For this review, take the finished solid that the model builds, in its own axes (mm). A direction names the side the tool comes from. Coordinates: 2 decimals unless noted, no trailing zeros. Loops run counter-clockwise (first coordinate to the right, second up) from the corner with the lowest first, then second, coordinate; pieces in that order, holes last. Notation, with made-up numbers: (-5, 22.25) - (12, 22.25) arc R11 cw to (12, 43.25) - close; hole circle Ø2 at (-16.75, 75). An arc over 180 degrees is marked (long way). Answer as a JSON object with one key per item and string values. Group by question number.
Item 1: Clearance check with flat-ended pins moving along their axes: pin 1 (1.8 mm diameter, centred on y = -4.5, z = -6, fed in from -X); pin 2 (3 mm diameter, centred on y = -2.5, z = -2.5, fed in from +X); pin 3 (1.5 mm diameter, centred on y = -2.5, z = -10.5, fed in from -X). State where each tip first meets the part, or that it passes through.
Item 2: Tool access review of faces 5 (the cylindrical face through (6.47, -3.46, 11.38)), 6 (the flat face through (2.5, -3, -2)): name each direction out of +Z, -Z, +X, -X, +Y, -Y from which nothing blocks a thin tool from reaching the whole face with its end or side.
Item 3: We need section B-B (x = 1.5). State how many separate pieces and enclosed holes the cut face has, then the cut area to 3 significant figures.
Item 4: We need section A-A (z = 1). Give the boundary of the cut face in (x, y), then the cut area to 3 significant figures.
Item 5: To check wall thickness, follow line 1 (X direction, y = -2, z = 10.75); line 2 (Z direction, x = -1.5, y = -1.5); line 3 (X direction, y = -2.75, z = 8). State the ranges of each line that lie inside material, in increasing order.
Item 6: Mouldability with a two-part tool opening along Z and no side actions: class faces 1 (the cylindrical face through (0.03, -1, -11.45)), 2 (the cylindrical face through (-6.47, -3.46, 11.38)), 3 (the cylindrical face through (-0.03, -2.96, -11.44)), 4 (the flat face through (-2.5, -3, -2)) as released by +Z, released by -Z, zero draft, split by the parting line, or undercut.
from build123d import *

# Parameters (mm, degrees)
F0_W         = 5
F0_H         = 17
F1_DEPTH     = 7
F3_D         = 5
F4_T1_DEPTH  = 29.5
F5_R         = 3.49999
F6_R         = 3
F7_T1_DEPTH  = 10.7715938526
F7_T3_DEPTH  = 7
F7_T5_DEPTH  = 2e-05
F7_T16_ANGLE = 74.5339900582
F7_T18_ANGLE = 117.281460121
F7_T20_ANGLE = 132.7531885059
F7_T22_ANGLE = 74.5339900582
F7_T24_ANGLE = 117.281460121
F7_T26_ANGLE = 132.7531885059
F7_T28_ANGLE = 90
F7_T30_ANGLE = 90
F7_T34_ANGLE = 74.5339900582
F7_T36_ANGLE = 90
F7_T38_ANGLE = 117.281460121
F7_T40_ANGLE = 90
F7_T44_ANGLE = 132.7531885059
F7_T46_ANGLE = 74.5339900582
F7_T48_ANGLE = 117.281460121
F7_T50_ANGLE = 132.7531885059


# Not quite as in the source:
# - a fillet or chamfer that OpenCascade refuses, or shapes differently, is made with other operations: its cross-section is extruded or revolved along the edge and cut away or added
# - two fillets or chamfers of one size are made in one step
# - a fillet or chamfer is up to 0.001 mm smaller than in the source, because OpenCascade refuses the exact size


with BuildPart() as f1:
    # F0 (on Front) → F1 (new body)
    with BuildSketch(Plane.XZ):
        with BuildLine():
            Line((8, 12.5), (2.5, 12.5))
            Line((2.5, 12.5), (2.5, 11.0980762114))
            ThreePointArc((2.5, 11.0980762114), (5.5, 11.0980762114), (7, 8.5))
            ThreePointArc((7, 8.5), (5.5, 5.9019237886), (2.5, 5.9019237886))
            Line((2.5, 5.9019237886), (2.5, 4.5))
            Line((2.5, 4.5), (8, 4.5))
            Line((8, 4.5), (8, 12.5))
        make_face()
        with BuildLine():
            Line((-2.5, 11.0980762114), (-2.5, 12.5))
            Line((-2.5, 12.5), (-8, 12.5))
            Line((-8, 12.5), (-8, 4.5))
            Line((-8, 4.5), (-2.5, 4.5))
            Line((-2.5, 4.5), (-2.5, 5.9019237886))
            ThreePointArc((-2.5, 5.9019237886), (-7, 8.5), (-2.5, 11.0980762114))
        make_face()
        with BuildLine():
            Line((2.5, 11.0980762114), (2.5, 12.5))
            Line((2.5, 12.5), (-2.5, 12.5))
            Line((-2.5, 12.5), (-2.5, 11.0980762114))
            ThreePointArc((-2.5, 11.0980762114), (-1.4019237886, 10), (-1, 8.5))
            ThreePointArc((-1, 8.5), (-1.4019237886, 7), (-2.5, 5.9019237886))
            Line((-2.5, 5.9019237886), (-2.5, 4.5))
            Line((-2.5, 4.5), (2.5, 4.5))
            Line((2.5, 4.5), (2.5, 5.9019237886))
            ThreePointArc((2.5, 5.9019237886), (1, 8.5), (2.5, 11.0980762114))
        make_face()
        with Locations((0, -4)):
            Rectangle(F0_W, F0_H)
    extrude(amount=F1_DEPTH)

    # F3 (through all)
    with Locations(Plane.YZ.offset(2.5)):
        with Locations((-3.5, -9)):
            Hole(F3_D / 2)

    # F4: fillet of radius 4.5 on 4 edges, made by hand

    # F4_s2 → F4_t1 (cut)
    with BuildSketch(Plane.XZ.offset(-11.25)):
        with BuildLine():
            ThreePointArc((3.5, 12.5), (6.6819805153, 11.1819805153), (8, 8))
            Line((8, 8), (8, 12.5))
            Line((8, 12.5), (3.5, 12.5))
        make_face()
        with BuildLine():
            ThreePointArc((-3.5, 12.5), (-6.6819805153, 11.1819805153), (-8, 8))
            Line((-8, 8), (-8, 12.5))
            Line((-8, 12.5), (-3.5, 12.5))
        make_face()
        with BuildLine():
            ThreePointArc((8, 9), (6.6819805153, 5.8180194847), (3.5, 4.5))
            Line((3.5, 4.5), (8, 4.5))
            Line((8, 4.5), (8, 9))
        make_face()
        with BuildLine():
            ThreePointArc((-8, 9), (-6.6819805153, 5.8180194847), (-3.5, 4.5))
            Line((-3.5, 4.5), (-8, 4.5))
            Line((-8, 4.5), (-8, 9))
        make_face()
    extrude(amount=F4_T1_DEPTH, mode=Mode.SUBTRACT)

    # F5 (radius 3.5 in the source; OpenCascade refuses exactly that, so slightly less here)
    f5_edges = [f1.edges().sort_by_distance(p)[0] for p in [
        (0, 0, -12.5),
        (0, -7, -12.5),
    ]]
    fillet(f5_edges, radius=F5_R)

    # F6
    f6_edges = [f1.edges().sort_by_distance(p)[0] for p in [
        (2.5, -3.5, 4.5),
        (-2.5, -3.5, 4.5),
    ]]
    fillet(f6_edges, radius=F6_R)

    # F7: chamfer of 0.5 on 30 edges, made by hand

    # F7_s2 → F7_t1 (cut)
    with BuildSketch(Plane.XY.offset(-9.00001)):
        Polygon((2, 0), (2.5, -0.5), (2.5, 0), align=None)
        Polygon((-2, 0), (-2.5, -0.5), (-2.5, 0), align=None)
        Polygon((2.5, -6.5), (2, -7), (2.5, -7), align=None)
        Polygon((-2.5, -6.5), (-2, -7), (-2.5, -7), align=None)
    extrude(amount=F7_T1_DEPTH, mode=Mode.SUBTRACT)

    # F7_s4 → F7_t3 (cut)
    with BuildSketch(Plane.YZ.offset(-3.5)):
        Polygon((0, 12), (-0.5, 12.5), (0, 12.5), align=None)
        Polygon((-6.5, 12.5), (-7, 12), (-7, 12.5), align=None)
    extrude(amount=F7_T3_DEPTH, mode=Mode.SUBTRACT)

    # F7_s6 → F7_t5 (cut)
    with BuildSketch(Plane.XZ.offset(3.49999)):
        Polygon((2.5, -12), (2, -12.5), (2.5, -12.5), align=None)
        Polygon((-2.5, -12), (-2, -12.5), (-2.5, -12.5), align=None)
    extrude(amount=F7_T5_DEPTH, mode=Mode.SUBTRACT)

    # F7_s7 → F7_t8 (revolve, cut)
    with BuildSketch(Plane.XY.offset(8.5)):
        Polygon((-1, -6.5), (-0.5, -7), (-1, -7), align=None)
    revolve(axis=Axis((-4, -7, 8.5), (0, 1, 0)), mode=Mode.SUBTRACT)

    # F7_s9 → F7_t10 (revolve, cut)
    with BuildSketch(Plane(origin=(-0.6806079661, 0, 0.3929491924), x_dir=(0, 1, 0), z_dir=(0.8660254038, 0, -0.5))):
        Polygon((-6.5, 6.3612159322), (-7, 5.8612159322), (-7, 6.3612159322), align=None)
    revolve(axis=Axis((4, -7, 8.5), (0, 1, 0)), mode=Mode.SUBTRACT)

    # F7_s11 → F7_t12 (revolve, cut)
    with BuildSketch(Plane.XY.offset(8.5)):
        Polygon((-0.5, 0), (-1, -0.5), (-1, 0), align=None)
    revolve(axis=Axis((-4, 0, 8.5), (0, 1, 0)), mode=Mode.SUBTRACT)

    # F7_s13 → F7_t14 (revolve, cut)
    with BuildSketch(Plane(origin=(-0.6806079661, 0, 0.3929491924), x_dir=(0, 1, 0), z_dir=(0.8660254038, 0, -0.5))):
        Polygon((0, 5.8612159322), (-0.5, 6.3612159322), (0, 6.3612159322), align=None)
    revolve(axis=Axis((4, 0, 8.5), (0, 1, 0)), mode=Mode.SUBTRACT)

    # F7_s15 → F7_t16 (revolve, cut)
    with BuildSketch(Plane.XY.offset(1.771583853)):
        Polygon((2, 0), (2.5000000001, -0.5), (2.5, 0), align=None)
    revolve(axis=Axis((5.4999999996, 0, 1.771583853), (0, 1, 0)), revolution_arc=F7_T16_ANGLE, mode=Mode.SUBTRACT)

    # F7_s17 → F7_t18 (revolve, cut)
    with BuildSketch(Plane(origin=(-2.8735542897, 0, 3.1088689023), x_dir=(0, 1, 0), z_dir=(-0.6787683205, 0, 0.7343524815))):
        Polygon((0, -12.6791485698), (-0.5, -13.1791485698), (0, -13.1791485698), align=None)
    revolve(axis=Axis((3.4999999999, 0, 9.0000000001), (0, 1, 0)), revolution_arc=F7_T18_ANGLE, mode=Mode.SUBTRACT)

    # F7_s19 → F7_t20 (revolve, cut)
    with BuildSketch(Plane.YZ.offset(3.4999999999)):
        Polygon((0, 12), (-0.5, 12.5), (0, 12.5), align=None)
    revolve(axis=Axis((3.4999999999, 0, 7.9999999999), (0, 1, 0)), revolution_arc=F7_T20_ANGLE, mode=Mode.SUBTRACT)

    # F7_s21 → F7_t22 (revolve, cut)
    with BuildSketch(Plane.XY.offset(1.771583853)):
        Polygon((-2, 0), (-2.5000000001, -0.5), (-2.5, 0), align=None)
    revolve(axis=Axis((-5.4999999996, 0, 1.771583853), (0, -1, 0)), revolution_arc=F7_T22_ANGLE, mode=Mode.SUBTRACT)

    # F7_s23 → F7_t24 (revolve, cut)
    with BuildSketch(Plane(origin=(-5.5642042783, 0, 1.5395362318), x_dir=(0, 1, 0), z_dir=(0.9637888196, 0, -0.2666666667))):
        Polygon((0, 3.7407660435), (-0.5, 3.2407660435), (0, 3.2407660435), align=None)
    revolve(axis=Axis((-3.4999999999, 0, 9.0000000001), (0, 1, 0)), revolution_arc=F7_T24_ANGLE, mode=Mode.SUBTRACT)

    # F7_s25 → F7_t26 (revolve, cut)
    with BuildSketch(Plane(origin=(-5.6005949978, 0, 6.0580131587), x_dir=(0, 1, 0), z_dir=(0.6788416095, 0, -0.7342847331))):
        Polygon((0, -1.1392636899), (-0.5, -1.6392636899), (0, -1.6392636899), align=None)
    revolve(axis=Axis((-3.4999999999, 0, 7.9999999999), (0, 1, 0)), revolution_arc=F7_T26_ANGLE, mode=Mode.SUBTRACT)

    # F7_s27 → F7_t28 (revolve, cut)
    with BuildSketch(Plane.XY.offset(-9.00001)):
        Polygon((2.5, -0.5), (2, 0), (2.5, 0), align=None)
    revolve(axis=Axis((2.5, -3.49999, -9.00001), (-1, 0, 0)), revolution_arc=F7_T28_ANGLE, mode=Mode.SUBTRACT)

    # F7_s29 → F7_t30 (revolve, cut)
    with BuildSketch(Plane.XY.offset(-9.00001)):
        Polygon((2.5, -6.5), (2, -7), (2.5, -7), align=None)
    revolve(axis=Axis((2.5, -3.50001, -9.00001), (1, 0, 0)), revolution_arc=F7_T30_ANGLE, mode=Mode.SUBTRACT)

    # F7_s31 → F7_t32 (revolve, cut)
    with BuildSketch(Plane.XY.offset(-9)):
        Polygon((2.5, -0.5), (2, -1), (2.5, -1), align=None)
    revolve(axis=Axis((2.5, -3.5, -9), (1, 0, 0)), mode=Mode.SUBTRACT)

    # F7_s33 → F7_t34 (revolve, cut)
    with BuildSketch(Plane.XY.offset(1.771583853)):
        Polygon((2.5000000001, -6.5), (2, -7), (2.5, -7), align=None)
    revolve(axis=Axis((5.4999999996, -7, 1.771583853), (0, 1, 0)), revolution_arc=F7_T34_ANGLE, mode=Mode.SUBTRACT)

    # F7_s35 → F7_t36 (revolve, cut)
    with BuildSketch(Plane.XY.offset(-9.00001)):
        Polygon((-2, 0), (-2.5, -0.5), (-2.5, 0), align=None)
    revolve(axis=Axis((-2.5, -3.49999, -9.00001), (-1, 0, 0)), revolution_arc=F7_T36_ANGLE, mode=Mode.SUBTRACT)

    # F7_s37 → F7_t38 (revolve, cut)
    with BuildSketch(Plane(origin=(-2.8735542897, 0, 3.1088689023), x_dir=(0, 1, 0), z_dir=(-0.6787683205, 0, 0.7343524815))):
        Polygon((-6.5, -13.1791485698), (-7, -12.6791485698), (-7, -13.1791485698), align=None)
    revolve(axis=Axis((3.4999999999, -7, 9.0000000001), (0, 1, 0)), revolution_arc=F7_T38_ANGLE, mode=Mode.SUBTRACT)

    # F7_s39 → F7_t40 (revolve, cut)
    with BuildSketch(Plane.XY.offset(-9.00001)):
        Polygon((-2.5, -6.5), (-2, -7), (-2.5, -7), align=None)
    revolve(axis=Axis((-2.5, -3.50001, -9.00001), (1, 0, 0)), revolution_arc=F7_T40_ANGLE, mode=Mode.SUBTRACT)

    # F7_s41 → F7_t42 (revolve, cut)
    with BuildSketch(Plane.XY.offset(-9)):
        Polygon((-2.5, -0.5), (-2, -1), (-2.5, -1), align=None)
    revolve(axis=Axis((-2.5, -3.5, -9), (1, 0, 0)), mode=Mode.SUBTRACT)

    # F7_s43 → F7_t44 (revolve, cut)
    with BuildSketch(Plane.YZ.offset(3.4999999999)):
        Polygon((-6.5, 12.5), (-7, 12), (-7, 12.5), align=None)
    revolve(axis=Axis((3.4999999999, -7, 7.9999999999), (0, 1, 0)), revolution_arc=F7_T44_ANGLE, mode=Mode.SUBTRACT)

    # F7_s45 → F7_t46 (revolve, cut)
    with BuildSketch(Plane.XY.offset(1.771583853)):
        Polygon((-2.5000000001, -6.5), (-2, -7), (-2.5, -7), align=None)
    revolve(axis=Axis((-5.4999999996, -7, 1.771583853), (0, -1, 0)), revolution_arc=F7_T46_ANGLE, mode=Mode.SUBTRACT)

    # F7_s47 → F7_t48 (revolve, cut)
    with BuildSketch(Plane(origin=(-5.5642042783, 0, 1.5395362318), x_dir=(0, 1, 0), z_dir=(0.9637888196, 0, -0.2666666667))):
        Polygon((-6.5, 3.2407660435), (-7, 3.7407660435), (-7, 3.2407660435), align=None)
    revolve(axis=Axis((-3.4999999999, -7, 9.0000000001), (0, 1, 0)), revolution_arc=F7_T48_ANGLE, mode=Mode.SUBTRACT)

    # F7_s49 → F7_t50 (revolve, cut)
    with BuildSketch(Plane(origin=(-5.6005949978, 0, 6.0580131587), x_dir=(0, 1, 0), z_dir=(0.6788416095, 0, -0.7342847331))):
        Polygon((-6.5, -1.6392636899), (-7, -1.1392636899), (-7, -1.6392636899), align=None)
    revolve(axis=Axis((-3.4999999999, -7, 7.9999999999), (0, 1, 0)), revolution_arc=F7_T50_ANGLE, mode=Mode.SUBTRACT)


solid = f1.part
Check sheet entries:
{
 "1": {"pin 1": "stops at x = -2.5", "pin 2": "stops at x = 2.5", "pin 3": "stops at x = -2.05"},
 "2": {"face 5": "+Z, +X, +Y, -Y", "face 6": "-Z, +X, +Y, -Y"},
 "3": {"separate pieces": "2", "enclosed holes": "1", "area": "126 mm2"},
 "4": {"outline": "(-2.5, -6.5) - (-2, -7) - (2, -7) - (2.5, -6.5) - (2.5, -0.5) - (2, 0) - (-2, 0) - (-2.5, -0.5) - close", "area": "34.5 mm2"},
 "5": {"line 1": "x = -7.06 to -5.98, -2.02 to 2.02, 5.98 to 7.06", "line 2": "z = -11.87 to -10.5, -7.5 to 6.84, 10.16 to 12.5", "line 3": "x = -7.89 to -6.96, -1.04 to 1.04, 6.96 to 7.89"},
 "6": {"face 1": "released by -Z", "face 2": "released by +Z", "face 3": "undercut", "face 4": "zero draft"}
}
